Verification items for the finished model (mm, model axes). Face numbers are marked on the shaded views. A direction names the side the tool comes from. Round coordinates to 2 decimals unless told otherwise and drop trailing zeros. Order: outer loops, then holes, each group sorted by start corner. A loop starts at its lowest first (then second) coordinate and runs counter-clockwise, first axis right, second up. Notation, with made-up numbers: (-25.75, 21.5) -> (-16.75, 21.5) arc R25 cw to (-16.75, 47.5) -> close; hole circle Ø11 at (42.5, -7.5). An arc over 180 degrees is marked (long way). Return JSON: item names as keys, results as strings. Group by question number.
1) Draft check along X on the marked faces 1, 2, 3 and 4. Enter one of: pulls with the +X half, pulls with the -X half, needs draft (parallel to the pull), parting line crosses it, or undercut.
2) Section check B-B on y = -27. Enter the section's corners in (x, z), plus the area to 3 significant figures.
3) Scan lines: L1, parallel to X at y = -19, z = 38; L2, parallel to Z at x = -48, y = -22; L3, parallel to Y at x = -43, z = 34. Record each from-to range of solid material in increasing order.
4) Tool access check on the marked faces 5, 6 and 7. Record the directions out of +Z, -Z, +X, -X, +Y, -Y that give a thin tool (end or side, any length) a straight path to the whole face; none if there is none.
5) Section check A-A on y = -17. Enter the section's corners in (x, z).
6) Depth check by flat-ended pin: pin 1 (4 mm diameter, centred on x = -31.5, y = -29.5, fed in from +Z); pin 2 (7.5 mm diameter, centred on x = -43.5, z = 39.5, fed in from +Y); pin 3 (6 mm diameter, centred on x = -58.5, z = 31, fed in from -Y). Enter the tip coordinate at first touch or a pass-through.
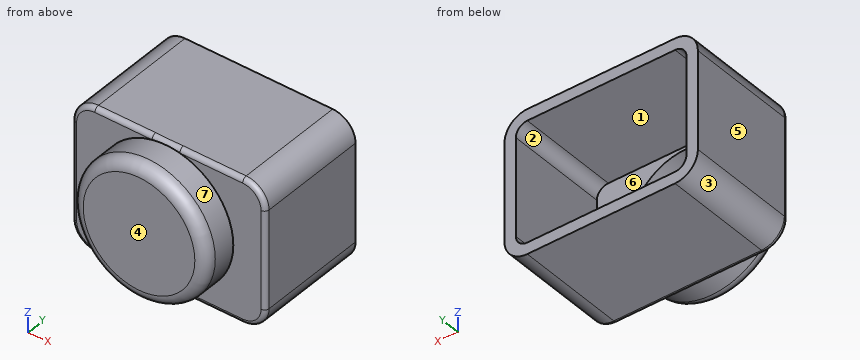
```python
from build123d import *

# Parameters (mm, degrees)
F0_W     = 42.9490916431
F0_H     = 31.8654570729
F1_DEPTH = 25.4
F2_R     = 5.08
F3_T     = -2.54
F4_R     = 14.9347335013
F5_DEPTH = 7.62
F6_R     = 2.54
F7_T     = 2.54
F8_R     = 1


# Not quite as in the source:
# - a shell that OpenCascade refuses in one call is made with other operations: the cavity is built on its own and cut out


with BuildPart() as f1:
    # F0 (on Front) → F1 (new body)
    with BuildSketch(Plane.XZ):
        with Locations((-42.025456205, 33.8281830773)):
            Rectangle(F0_W, F0_H)
    extrude(amount=F1_DEPTH)

    # F2
    f2_edges = [f1.edges().sort_by_distance(p)[0] for p in [
        (-63.500002, -12.7, 49.760912),
        (-20.55091, -12.7, 49.760912),
        (-20.55091, -12.7, 17.895455),
        (-63.500002, -12.7, 17.895455),
    ]]
    fillet(f2_edges, radius=F2_R)

    # F3
    f3_openings = [f1.faces().sort_by_distance(p)[0] for p in [
        (-42.025456, 0, 33.828183),
    ]]
    offset(amount=F3_T, openings=f3_openings)

    # F4 (on face) → F5 (join)
    with BuildSketch(Plane.XZ.offset(25.4)):
        with Locations((-42.6500104368, 34.1481156647)):
            Circle(F4_R)
    extrude(amount=F5_DEPTH)

    # F6
    f6_edges = [f1.edges().sort_by_distance(p)[0] for p in [
        (-57.584744, -33.02, 34.148116),
    ]]
    fillet(f6_edges, radius=F6_R)

    # F7: shell of thickness 2.54, made by hand


with BuildPart() as f7_core1:
    # F7_t2: copy of F1
    add(f1.part)

    # the walls: a layer under each face that stays
    f7_faces = [f7_core1.faces().sort_by_distance(p)[0] for p in [
        (-57.5847439381, -27.94, 34.1481156647),
        (-56.341820086, -25.4, 23.206364053),
        (-42.6500104368, -33.02, 34.1481156647),
        (-42.025456205, -12.7, 49.7609116137),
        (-22.038807935, -12.7, 48.2730140621),
        (-62.012104475, -12.7, 48.2730140621),
        (-20.5509103835, -12.7, 33.8281830773),
        (-63.5000020266, -12.7, 33.8281830773),
        (-22.038807935, -12.7, 19.3833520924),
        (-62.012104475, -12.7, 19.3833520924),
        (-42.025456205, -12.7, 17.8954545408),
        (-60.4322097663, 0, 20.1715586175),
        (-42.025456205, -11.43, 47.2209116137),
        (-23.8348591592, -11.43, 46.4769628379),
        (-23.0909103835, -11.43, 33.8281830773),
        (-23.8348591592, -11.43, 21.1794033166),
        (-42.025456205, -11.43, 20.4354545408),
        (-60.2160532508, -11.43, 21.1794033166),
        (-60.9600020266, -11.43, 33.8281830773),
        (-60.2160532508, -11.43, 46.4769628379),
    ]]
    thicken(f7_faces, amount=-F7_T, mode=Mode.SUBTRACT)

    # F7_s3 → F7_t4 (revolve, cut)
    with BuildSketch(Plane.XY.offset(34.1481156647)):
        Polygon((-27.6898769355, -25.4254), (-30.2552769355, -25.4), (-30.2552769355, -22.86), (-27.7152769355, -22.86), align=None)
    revolve(axis=Axis((-42.6500104368, -25.4, 34.1481156647), (0, -1, 0)), mode=Mode.SUBTRACT)


with BuildPart() as f1_1:
    add(f1.part)

    # what is left inside the walls is the cavity
    f7_cavity = [f7_core1.part.solids().sort_by_distance(p)[0] for p in [
        (-55.019344, -27.94, 34.148116),
    ]]
    add(f7_cavity, mode=Mode.SUBTRACT)

    # F8
    f8_edges = [f1_1.edges().sort_by_distance(p)[0] for p in [
        (-42.025456, -25.4, 49.760912),
        (-22.038808, -25.4, 48.273014),
        (-62.012104, -25.4, 48.273014),
        (-20.55091, -25.4, 33.828183),
        (-63.500002, -25.4, 33.828183),
        (-22.038808, -25.4, 19.383352),
        (-62.012104, -25.4, 19.383352),
        (-42.025456, -25.4, 17.895455),
    ]]
    fillet(f8_edges, radius=F8_R)


solid = f1_1.part
```
Check result:
{
 "1": {"face 1": "undercut", "face 2": "undercut", "face 3": "pulls with the -X half", "face 4": "needs draft"},
 "2": {"outline": "circle Ø29.87 at (-42.65, 34.15); hole circle Ø24.79 at (-42.65, 34.15)", "area": "218 mm^2"},
 "3": {"L1": "-63.5 to -60.96, -23.09 to -20.55", "L2": "17.9 to 20.44, 47.22 to 49.76", "L3": "-33.02 to -30.48"},
 "4": {"face 5": "+Z, -Z, -X, +Y, -Y", "face 6": "+Y", "face 7": "-Y"},
 "5": {"outline": "(-63.5, 22.98) arc R5.08 ccw to (-58.42, 17.9) -> (-25.63, 17.9) arc R5.08 ccw to (-20.55, 22.98) -> (-20.55, 44.68) arc R5.08 ccw to (-25.63, 49.76) -> (-58.42, 49.76) arc R5.08 ccw to (-63.5, 44.68) -> close; hole (-60.96, 22.98) arc R2.54 ccw to (-58.42, 20.44) -> (-25.63, 20.44) arc R2.54 ccw to (-23.09, 22.98) -> (-23.09, 44.68) arc R2.54 ccw to (-25.63, 47.22) -> (-58.42, 47.22) arc R2.54 ccw to (-60.96, 44.68) -> close"},
 "6": {"pin 1": "z = 45.95", "pin 2": "y = -30.48", "pin 3": "y = -32.9"}
}
